Autodesk Inventor part; units mm, degrees
ref_plane "YZ Plane" through (0, 0, 0) normal (1, 0, 0) x (0, 1, 0)
ref_plane "XZ Plane" through (0, 0, 0) normal (0, 1, 0) x (-1, 0, 0)
ref_plane "XY Plane" through (0, 0, 0) normal (0, 0, 1) x (1, 0, 0)
ref_plane "Arbeitsebene1" through (0, 0, 0) normal (0, 0, 1) x (1, 0, 0)
sketch "Skizze1" plane through (0, 0, 0) normal (0, 0, 1) x (1, 0, 0)
  arc A0 (63, -2) -> (61, 0) centre (61, -2) ccw
  line L0 (61, 0) -> (60, 0)
  line L1 (60, 0) -> (60, -30)
  line L2 (60, -30) -> (-40, -30)
  line L3 (-40, -30) -> (-40, 40)
  line L4 (-40, 40) -> (60, 40)
  line L5 (60, 40) -> (60, 10)
  line L6 (60, 10) -> (61, 10)
  arc A1 (61, 10) -> (63, 12) centre (61, 12) ccw
  line L7 (63, 12) -> (63, 41)
  arc A2 (63, 41) -> (61, 43) centre (61, 41) ccw
  line L8 (61, 43) -> (-41, 43)
  arc A3 (-41, 43) -> (-43, 41) centre (-41, 41) ccw
  line L9 (-43, 41) -> (-43, -31)
  arc A4 (-43, -31) -> (-41, -33) centre (-41, -31) ccw
  line L10 (-41, -33) -> (61, -33)
  arc A5 (61, -33) -> (63, -31) centre (61, -31) ccw
  line L11 (63, -31) -> (63, -2)
  line L12 (63, 12) -> (63, -2)
  point P0 (0, 0)
extrude "Extrusion1" add sketch "Skizze1" along normal blind 3
sketch "Skizze2" plane through (0, 0, 0) normal (0, 0, -1) x (-1, 0, 0)
  line L0 (40, -30) -> (-60, -30) construction
  line L1 (-60, -30) -> (-60, 40) construction
  line L2 (-60, 40) -> (40, 40) construction
  line L3 (40, 40) -> (40, -30) construction
  line L4 (40, -24.5) -> (37, -24.5)
  line L5 (37, -24.5) -> (37, -19.5)
  line L6 (37, -19.5) -> (40, -19.5)
  line L7 (40, -19.5) -> (40, -24.5)
  line L8 (40, 29.5) -> (37, 29.5)
  line L9 (37, 29.5) -> (37, 34.5)
  line L10 (37, 34.5) -> (40, 34.5)
  line L11 (40, 34.5) -> (40, 29.5)
  line L12 (-60, -24.5) -> (-57, -24.5)
  line L13 (-57, -24.5) -> (-57, -19.5)
  line L14 (-57, -19.5) -> (-60, -19.5)
  line L15 (-60, -19.5) -> (-60, -24.5)
  line L16 (-60, 29.5) -> (-57, 29.5)
  line L17 (-57, 29.5) -> (-57, 34.5)
  line L18 (-57, 34.5) -> (-60, 34.5)
  line L19 (-60, 34.5) -> (-60, 29.5)
  line L20 (37, -22) -> (40, -22) construction
  line L21 (37, 32) -> (40, 32) construction
  point P0 (38.5, -22)
  dimension "d2" = 3
  dimension "d3" = 5
  dimension "d4" = 8
  dimension "d5" = 8
extrude "Extrusion2" add sketch "Skizze2" along normal blind 6
sketch "Skizze4" plane through (0, 0, 0) normal (0, 0, -1) x (-1, 0, 0)
  line L0 (-60, 40) -> (40, 40)
  line L1 (40, -30) -> (-60, -30)
  line L2 (-9.7574, 40) -> (-9.7574, 38)
  line L3 (-9.7574, 38) -> (-29.7574, 38)
  line L4 (-29.7574, 38) -> (-29.7574, 40)
  line L5 (-9.7574, -30) -> (-9.7574, -28)
  line L6 (-9.7574, -28) -> (-29.7574, -28)
  line L7 (-29.7574, -28) -> (-29.7574, -30)
  point P0 (0, 0)
  dimension "d10" = 2
  dimension "d11" = 20
extrude "Extrusion3" add sketch "Skizze4" along normal blind 2
fillet "Rundung1" radius 4 8 edges at (-38.5, 34.5, 0) (-38.5, 29.5, 0) (-38.5, -24.5, 0) (-38.5, -19.5, 0) (58.5, 34.5, 0) (58.5, -19.5, 0) (58.5, 29.5, 0) (58.5, -24.5, 0)
sketch "Skizze5" plane through (60, 29.5, -6) normal (1, 0, 0) x (0, 0, -1)
  circle A0 centre (-3, 2.5) radius 1.55
  circle A1 centre (-3, -51.5) radius 1.55
  point P0 (-6, -29.5)
extrude "Extrusion4" cut sketch "Skizze5" against normal through all
fillet "Rundung2" radius 2 8 edges at (58.5, 29.5, -6) (58.5, 34.5, -6) (58.5, -24.5, -6) (58.5, -19.5, -6) (-38.5, 29.5, -6) (-38.5, 34.5, -6) (-38.5, -24.5, -6) (-38.5, -19.5, -6)
properties part number "Box_Arduino_Oben_2"
Could you check a few things on this model? Use its own coordinates, in mm. A direction names the side the tool comes from. Coordinates: 2 decimals unless noted, no trailing zeros. Order: outer loops, then holes, each group sorted by start corner. A loop starts at its lowest first (then second) coordinate and runs counter-clockwise, first axis right, second up. Notation, with made-up numbers: (-8.5, 56) -> (21.5, 56) arc R24 ccw to (21.5, 78) -> close; hole circle Ø3 at (-37.75, 39.5). An arc over 180 degrees is marked (long way). One line per item, written item: value. Start each with the question number.
1) We'd pull the mould along X, two halves only. Please class faces 1 (the flat face through (57, 32, -1)), 2 (the cylindrical face through (-42.43, 42.4, 1.48)), 3 (the flat face through (9, 6, 3)): +X half, -X half, draft (parallel to the pull), parting line (faces both ways), or undercut.
2) If I drill on L1, parallel to Y at x = -39, z = -3; L2, parallel to Z at x = -13, y = 13, over which ranges is the centre line in solid material (lowest first)? Write a range as [from, to].
3) Imagine slicing it at C-C on y = -18. List the corners of the cut face in (x, z) for me.
4) Imagine slicing it at D-D on y = -9.5. List the corners of the cut face in (x, z) for me.
5) I'm going to push flat-ended pins straight in: pin 1 (1.8 mm diameter, centred on y = -25, z = -4, fed in from +X); pin 2 (8 mm diameter, centred on x = 2.5, y = -6, fed in from -Z); pin 3 (1.6 mm diameter, centred on y = 39, z = -1, fed in from +X). Where does each tip first touch, or does it pass through?
6) Which directions (+Z, -Z, +X, -X, +Y, -Y) give clear straight access to the entire face, cutting with the end or side of a thin tool? Please do faces 4 (the flat face through (-40, 32, -1)), 5 (the flat face through (-37, -22, -1)), 6 (the cylindrical face through (-38.479, 28.359, -1.203)), 7 (the flat face through (20, 39, -2)), 8 (the flat face through (20, 40, -1)).
7) Imagine slicing it at A-A on y = 27. List the corners of the cut face in (x, z) for me.
8) Imagine slicing it at B-B on x = -2.5. List the corners of the cut face in (y, z) for me, plus the area to 3 significant figures.
Answer list:
1. face 1: undercut
1. face 2: -X half
1. face 3: draft
2. L1: y = [-24.63, -23.55], [-20.45, -19.37], [29.37, 30.45], [33.55, 34.63]
2. L2: z = [0, 3]
3. outline: (-43, 0) -> (-40, 0) -> (-40, -0.88) -> (-37, -0.88) -> (-37, 0) -> (57, 0) -> (57, -0.88) -> (60, -0.88) -> (60, 0) -> (63, 0) -> (63, 3) -> (-43, 3) -> close
4. outline: (-43, 0) -> (63, 0) -> (63, 3) -> (-43, 3) -> close
5. pin 1: stops at x = 60
5. pin 2: stops at z = 0
5. pin 3: stops at x = 29.76
6. face 4: -Z, -X, +Y, -Y
6. face 5: -Z, +Y, -Y
6. face 6: -Z, +X, -X
6. face 7: -Z, +X, -X, +Y, -Y
6. face 8: -Z, +X, -X, +Y
7. outline: (-43, 0) -> (-40, 0) -> (-40, -0.29) -> (-37, -0.29) -> (-37, 0) -> (57, 0) -> (57, -0.29) -> (60, -0.29) -> (60, 0) -> (63, 0) -> (63, 3) -> (-43, 3) -> close
8. outline: (-33, 0) -> (43, 0) -> (43, 3) -> (-33, 3) -> close
8. area: 228 mm2
